Check sheet for the modelled part. Datum: model origin and axes. Units: mm. A direction names the side the tool comes from. Coordinates: 2 decimals unless noted, no trailing zeros. Loops run counter-clockwise (first coordinate to the right, second up) from the corner with the lowest first, then second, coordinate; pieces in that order, holes last.
from build123d import *

# Parameters (mm, degrees)
F_1_8_0_125_DIAMETER_HOLE1_D   = 3.175
F_1_8_START                    = -4.7625001
F_1_8_0_1250_DOWEL_SLOT1_DEPTH = 9.5250001


# Read off the part's stored shape, not the designer's step: 1/8 (0.1250) Dowel Slot1
with BuildPart() as part:
    # Sketch1 → Revolve1 (revolve)
    with BuildSketch(Plane.XY, mode=Mode.PRIVATE) as revolve1_sk:
        Polygon((-18.8585, 0), (18.8585, 0), (18.8585, 5.1181), (16.3185, 5.1181), (16.3185, 3.0861), (12.7625, 3.0861), (12.7625, 5.1181), (10.2225, 5.1181), (10.2225, 3.0861), (6.6665, 3.0861), (6.6665, 5.1181), (-2.8585, 5.1181), (-2.8585, 4.7625), (-18.8585, 4.7625), align=None)
    revolve(revolve1_sk.sketch.rotate(Axis((-18.8585, 0, 0), (1, 0, 0)), 180), axis=Axis((-18.8585, 0, 0), (1, 0, 0)))

    # 1/8 (0.125) Diameter Hole1 (through all)
    with Locations(Plane(origin=(0, -5.1181, 0), x_dir=(-1, 0, 0), z_dir=(0, -1, 0))):
        with Locations((-1.904, 0)):
            Hole(F_1_8_0_125_DIAMETER_HOLE1_D / 2)

    # 1/8 (0.1250) Dowel Slot1 outline → 1/8 (0.1250) Dowel Slot1 (cut)
    with BuildSketch(Plane(origin=(0, 0, 0), x_dir=(1, 0, 0), z_dir=(0, 1, 0)).offset(F_1_8_START)):
        with BuildLine():
            ThreePointArc((-9.271, 0.499999), (-10.8585, 2.087499), (-12.446, 0.499999))
            Line((-12.446, 0.499999), (-12.446, -0.499999))
            ThreePointArc((-12.446, -0.499999), (-10.8585, -2.087499), (-9.271, -0.499999))
            Line((-9.271, -0.499999), (-9.271, 0.499999))
        make_face()
    extrude(amount=F_1_8_0_1250_DOWEL_SLOT1_DEPTH, mode=Mode.SUBTRACT)


solid = part.part
(1) Set-up check for faces 1 (the face through (-9.271, 0, 0)), 2 (the face through (-10.97, 3.78, 2.9)), 3 (the face through (10.222, 0.1, 3.3)), 4 (the face through (1.84, -4.73, 1.96)): record each of +Z, -Z, +X, -X, +Y, -Y from which the full face is reachable in a straight line by a thin tool's end or side.
(2) Draft check along X on faces 5 (the face through (18.858, 0, 0)), 6 (the face through (8.42, 2.449, 1.878)), 7 (the face through (17.571, 4.062, 3.114)). Enter one of: pulls with the +X half, pulls with the -X half, needs draft (parallel to the pull), parting line crosses it, or undercut.
(3) Section check B-B, the plane y = 4. Enter the section's corners in (x, z) (1 decimal), plus the area to 3 significant figures.
(4) Section check A-A, the plane z = 0. Count the separate pieces of the cut face and the enclosed holes in it, plus the area to 3 significant figures.
(5) Gauge pin test, flat ends, axial feed: P1, Ø4, axis at x = -13, z = 3, coming from the +Y side; P2, Ø5, axis at x = 4.5, y = 2, coming from the -Z side; P3, Ø5, axis at x = -6, z = 1.5, coming from the -Y side; P4, Ø1.5, axis at x = -12.5, z = -3.5, coming from the +Y side. Record the tip position at first contact, or that the pin passes through.
(6) Section check D-D, the plane x = -6. Enter the section's corners in (y, z) (1 decimal).
(7) Scan lines: line 1 along X through (y, z) = (-1.5, -0.75); line 2 along X through (y, z) = (3.25, -1.25); line 3 along X through (y, z) = (-4, -0.75). Record each from-to range of solid material in increasing order.
Determined:
1. face 1: +Y, -Y
1. face 2: -X
1. face 3: none
1. face 4: +X, -X
2. face 5: pulls with the +X half
2. face 6: undercut
2. face 7: needs draft
3. outline: (-18.9, -2.6) - (-2.9, -2.6) - (-2.9, -3.2) - (6.7, -3.2) - (6.7, 3.2) - (-2.9, 3.2) - (-2.9, 2.6) - (-18.9, 2.6) - close; (10.2, -3.2) - (12.8, -3.2) - (12.8, 3.2) - (10.2, 3.2) - close; (16.3, -3.2) - (18.9, -3.2) - (18.9, 3.2) - (16.3, 3.2) - close; hole (-12.4, -0.5) arc R1.6 ccw to (-9.3, -0.5) - (-9.3, 0.5) arc R1.6 ccw to (-12.4, 0.5) - close; hole circle Ø3.2 at (1.9, 0)
3. area: 157 mm2
4. separate pieces: 3
4. enclosed holes: 0
4. area: 283 mm2
5. P1: stops at y = 4.66
5. P2: stops at z = -5.12
5. P3: stops at y = -4.76
5. P4: stops at y = 3.89
6. outline: circle Ø9.5 at (0, 0)
7. line 1: x = -18.86 to -12.43, -9.29 to 0.5, 3.3 to 18.86
7. line 2: x = -18.86 to -12.26, -9.46 to 0.93, 2.88 to 6.67, 10.22 to 12.76, 16.32 to 18.86
7. line 3: x = -18.86 to -12.43, -9.29 to 0.5, 3.3 to 6.67, 10.22 to 12.76, 16.32 to 18.86
